Geometry check sheet. Reference: the model listing, model coordinates, mm. A direction names the side the tool comes from. Give positions to 0.01 mm unless a question says otherwise; leave off trailing zeros. Loops run counter-clockwise (first coordinate to the right, second up) from the corner with the lowest first, then second, coordinate; pieces in that order, holes last. Notation, with made-up numbers: (-34, -14.75) -> (-25, -14.75) arc R31 ccw to (-25, 20.25) -> close; hole circle Ø11 at (4.5, -35.75). An arc over 180 degrees is marked (long way). One line per question, with ' | ' between items.
from build123d import *

# Parameters (mm, degrees)
F0_W     = 5.08
F0_H     = 5.08
F0_R     = 1.27
F0_W_2   = 53.340002
F0_H_2   = 58.42
F0_W_3   = 5.079998
F0_H_3   = 12.7
F1_DEPTH = 5.08


with BuildPart() as f1:
    # F0 (on Top) → F1 (new body)
    with BuildSketch(Plane.XY):
        with Locations((-38.3377, 31.580215)):
            Rectangle(F0_W, F0_H)
        with Locations((-38.3377, 31.580215)):
            Circle(F0_R, mode=Mode.SUBTRACT)
        with Locations((-9.127699, 31.580215)):
            Rectangle(F0_W_2, F0_H)
        with Locations((-38.3377, -0.169785)):
            Rectangle(F0_W, F0_H_2)
        with Locations((20.082301, 31.580215)):
            Rectangle(F0_W_3, F0_H)
        with Locations((20.082301, 31.580215)):
            Circle(F0_R, mode=Mode.SUBTRACT)
        with Locations((-38.3377, -35.729785)):
            Rectangle(F0_W, F0_H_3)
        with Locations((-38.3377, -39.031785)):
            Circle(F0_R, mode=Mode.SUBTRACT)
        with Locations((20.082301, -0.169785)):
            Rectangle(F0_W_3, F0_H_2)
        with Locations((-9.127699, -35.729785)):
            Rectangle(F0_W_2, F0_H_3)
        with Locations((20.082301, -35.729785)):
            Rectangle(F0_W_3, F0_H_3)
        with Locations((20.313209, -39.308877)):
            Circle(F0_R, mode=Mode.SUBTRACT)
    extrude(amount=F1_DEPTH)


solid = f1.part
Item 1: Set-up check for faces 1 (the face through (-9, 34.12, 3)), 2 (the face through (17.542, -1, 3)): record each of +Z, -Z, +X, -X, +Y, -Y from which the full face is reachable in a straight line by a thin tool's end or side.
Result:
face 1: +Z, -Z, +X, -X, +Y | face 2: +Z, -Z
Item 2: Sectioned sample at A-A (y = 27). Record the cut outline in (x, z).
Result:
outline: (-40.88, 0) -> (-35.8, 0) -> (-35.8, 5.08) -> (-40.88, 5.08) -> close; (17.54, 0) -> (22.62, 0) -> (22.62, 5.08) -> (17.54, 5.08) -> close
Item 3: Sectioned sample at B-B (x = -12.5). Record the cut outline in (y, z).
Result:
outline: (-42.08, 0) -> (-29.38, 0) -> (-29.38, 5.08) -> (-42.08, 5.08) -> close; (29.04, 0) -> (34.12, 0) -> (34.12, 5.08) -> (29.04, 5.08) -> close
Item 4: Sectioned sample at C-C (z = 1.25). Record the cut outline in (x, y), plus the area to 3 significant figures.
Result:
outline: (-40.88, -42.08) -> (22.62, -42.08) -> (22.62, 34.12) -> (-40.88, 34.12) -> close; hole circle Ø2.54 at (-38.34, -39.03); hole circle Ø2.54 at (-38.34, 31.58); hole (-35.8, -29.38) -> (17.54, -29.38) -> (17.54, 29.04) -> (-35.8, 29.04) -> close; hole circle Ø2.54 at (20.08, 31.58); hole circle Ø2.54 at (20.31, -39.31) | area: 1,700 mm2
Item 5: Scan lines: probe 1 along X at (y, z) = (0, 2.25); probe 2 along Y at (x, z) = (9, 2). Record each from-to range of solid material in increasing order.
Result:
probe 1: -40.88 to -35.8, 17.54 to 22.62 | probe 2: -42.08 to -29.38, 29.04 to 34.12
